The model under review builds one solid part; all positions refer to its coordinate system, in mm. Face numbers are marked on the shaded views. Round coordinates to 2 decimals unless told otherwise and drop trailing zeros. Write each loop counter-clockwise with the first axis right and the second up, starting at its lowest first coordinate (ties: lowest second). Pieces come first, ordered by that corner, then holes. Notation, with made-up numbers: (-22.5, 28) - (32.5, 28) arc R30 ccw to (32.5, 61) - close; hole circle Ø7 at (30, 40). An arc over 180 degrees is marked (long way). Use one line per item in the form item = value.
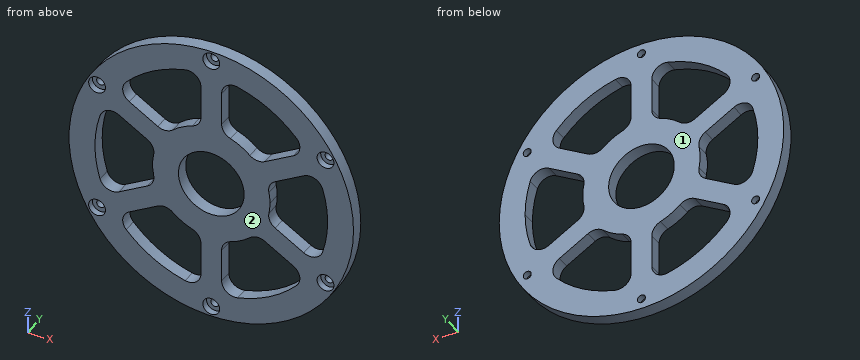
from build123d import *

# Parameters (mm, degrees)
SKETCH1_R           = 55
BOSS_EXTRUDE1_DEPTH = 5
SKETCH2_R           = 1.55
CUT_EXTRUDE1_DEPTH  = 6
SKETCH5_R           = 12.7
CUT_EXTRUDE4_DEPTH  = 6
CUT_EXTRUDE5_DEPTH  = 6
FILLET1_R           = 5
FILLET2_R           = 5
SKETCH8_R           = 3.25
CUT_EXTRUDE6_DEPTH  = 2.5
CIRPATTERN3_COUNT   = 6


with BuildPart() as part:
    # Sketch1 → Boss-Extrude1 (new body)
    with BuildSketch(Plane(origin=(0, 0, 0), x_dir=(1, 0, 0), z_dir=(0, 1, 0))):
        Circle(SKETCH1_R)
    extrude(amount=BOSS_EXTRUDE1_DEPTH)

    # Sketch2 → Cut-Extrude1 (cut, through all)
    with BuildSketch(Plane(origin=(0, 5, 0), x_dir=(1, 0, 0), z_dir=(0, 1, 0))):
        with Locations((0, 51)):
            Circle(SKETCH2_R)
        with Locations((44.167295593, 25.5)):
            Circle(SKETCH2_R)
        with Locations((44.167295593, -25.5)):
            Circle(SKETCH2_R)
        with Locations((0, -51)):
            Circle(SKETCH2_R)
        with Locations((-44.167295593, -25.5)):
            Circle(SKETCH2_R)
        with Locations((-44.167295593, 25.5)):
            Circle(SKETCH2_R)
    extrude(amount=-CUT_EXTRUDE1_DEPTH, mode=Mode.SUBTRACT)

    # Sketch5 → Cut-Extrude4 (cut, through all)
    with BuildSketch(Plane(origin=(0, 5, 0), x_dir=(1, 0, 0), z_dir=(0, 1, 0))):
        Circle(SKETCH5_R)
    extrude(amount=-CUT_EXTRUDE4_DEPTH, mode=Mode.SUBTRACT)

    # Sketch7 → Cut-Extrude5 (cut, through all)
    with BuildSketch(Plane(origin=(0, 5, 0), x_dir=(1, 0, 0), z_dir=(0, 1, 0))):
        with BuildLine():
            Line((-21.351162756, 7.708297411), (-40.816877772, 18.946833216))
            ThreePointArc((-40.816877772, 18.946833216), (-45, 0), (-40.816877772, -18.946833216))
            Line((-40.816877772, -18.946833216), (-21.351162756, -7.708297411))
            ThreePointArc((-21.351162756, -7.708297411), (-22.7, 0), (-21.351162756, 7.708297411))
        make_face()
        with BuildLine():
            Line((-17.351162756, -14.636500641), (-36.816877772, -25.875036446))
            ThreePointArc((-36.816877772, -25.875036446), (-22.5, -38.97114317), (-4, -44.821869662))
            Line((-4, -44.821869662), (-4, -22.344798052))
            ThreePointArc((-4, -22.344798052), (-11.35, -19.658776666), (-17.351162756, -14.636500641))
        make_face()
        with BuildLine():
            ThreePointArc((4, -44.821869662), (22.5, -38.97114317), (36.816877772, -25.875036446))
            Line((36.816877772, -25.875036446), (17.351162756, -14.636500641))
            ThreePointArc((17.351162756, -14.636500641), (11.35, -19.658776666), (4, -22.344798052))
            Line((4, -22.344798052), (4, -44.821869662))
        make_face()
        with BuildLine():
            ThreePointArc((45, 0), (43.941776818, 9.701559159), (40.816877772, 18.946833216))
            Line((40.816877772, 18.946833216), (21.351162756, 7.708297411))
            ThreePointArc((21.351162756, 7.708297411), (22.360248149, 3.912710406), (22.7, 0))
            ThreePointArc((22.7, 0), (22.360248149, -3.912710406), (21.351162756, -7.708297411))
            Line((21.351162756, -7.708297411), (40.816877772, -18.946833216))
            ThreePointArc((40.816877772, -18.946833216), (43.941776818, -9.701559159), (45, 0))
        make_face()
        with BuildLine():
            ThreePointArc((36.816877772, 25.875036446), (22.5, 38.97114317), (4, 44.821869662))
            Line((4, 44.821869662), (4, 22.344798052))
            ThreePointArc((4, 22.344798052), (11.35, 19.658776666), (17.351162756, 14.636500641))
            Line((17.351162756, 14.636500641), (36.816877772, 25.875036446))
        make_face()
        with BuildLine():
            Line((-4, 22.344798052), (-4, 44.821869662))
            ThreePointArc((-4, 44.821869662), (-22.5, 38.97114317), (-36.816877772, 25.875036446))
            Line((-36.816877772, 25.875036446), (-17.351162756, 14.636500641))
            ThreePointArc((-17.351162756, 14.636500641), (-11.35, 19.658776666), (-4, 22.344798052))
        make_face()
    extrude(amount=-CUT_EXTRUDE5_DEPTH, mode=Mode.SUBTRACT)

    # Fillet1
    fillet1_edges = [part.edges().sort_by_distance(p)[0] for p in [
        (-40.816877772, 2.5, -18.946833216),
        (-21.351162756, 2.5, -7.708297411),
        (-21.351162756, 2.5, 7.708297411),
        (-40.816877772, 2.5, 18.946833216),
    ]]
    fillet(fillet1_edges, radius=FILLET1_R)

    # Fillet2
    fillet2_edges = [part.edges().sort_by_distance(p)[0] for p in [
        (40.816877772, 2.5, 18.946833216),
        (21.351162756, 2.5, 7.708297411),
        (21.351162756, 2.5, -7.708297411),
        (40.816877772, 2.5, -18.946833216),
        (36.816877772, 2.5, -25.875036446),
        (17.351162756, 2.5, -14.636500641),
        (4, 2.5, -22.344798052),
        (4, 2.5, -44.821869662),
        (4, 2.5, 44.821869662),
        (4, 2.5, 22.344798052),
        (17.351162756, 2.5, 14.636500641),
        (36.816877772, 2.5, 25.875036446),
        (-36.816877772, 2.5, 25.875036446),
        (-17.351162756, 2.5, 14.636500641),
        (-4, 2.5, 22.344798052),
        (-4, 2.5, 44.821869662),
        (-4, 2.5, -44.821869662),
        (-4, 2.5, -22.344798052),
        (-17.351162756, 2.5, -14.636500641),
        (-36.816877772, 2.5, -25.875036446),
    ]]
    fillet(fillet2_edges, radius=FILLET2_R)

    # Sketch8 → Cut-Extrude6 (cut)
    with BuildSketch(Plane(origin=(0, 0, 0), x_dir=(1, 0, 0), z_dir=(0, 1, 0))):
        with Locations((0, 51)):
            Circle(SKETCH8_R)
    cut_extrude6 = extrude(amount=CUT_EXTRUDE6_DEPTH, mode=Mode.SUBTRACT)

    # CirPattern3: Cut-Extrude6 ×6 about axis
    cirpattern3_axis = Axis((0, 0, 0), (0, 1, 0))
    for i in range(1, CIRPATTERN3_COUNT):
        add(cut_extrude6.rotate(cirpattern3_axis, i * 360 / CIRPATTERN3_COUNT), mode=Mode.SUBTRACT)


solid = part.part
(1) Add section B-B on z = -1.5. Write out the cut boundary in (x, y) (3 decimals).
Geometry results:
outline = (-54.98, 0) - (-44.975, 0) - (-44.975, 5) - (-54.98, 5) - close; (-22.65, 0) - (-12.611, 0) - (-12.611, 5) - (-22.65, 5) - close; (12.611, 0) - (22.65, 0) - (22.65, 5) - (12.611, 5) - close; (44.975, 0) - (54.98, 0) - (54.98, 5) - (44.975, 5) - close
(2) To check wall thickness, follow L1, parallel to Z at x = 0, y = 4.05; L2, parallel to Z at x = 0, y = 0.7; L3, parallel to X at y = 1.7, z = -25.5. State the ranges of each line that lie inside material, in increasing order.
Geometry results:
L1 = -55 to -52.55, -49.45 to -12.7, 12.7 to 49.45, 52.55 to 55
L2 = -55 to -54.25, -47.75 to -12.7, 12.7 to 47.75, 54.25 to 55
L3 = -48.73 to -47.42, -40.92 to -33.92, -4.05 to 4.05, 33.92 to 40.92, 47.42 to 48.73
(3) Add section C-C on z = 51. Write out the cut boundary in (x, y).
Geometry results:
outline = (-20.59, 0) - (-3.25, 0) - (-3.25, 2.5) - (-1.55, 2.5) - (-1.55, 5) - (-20.59, 5) - close; (1.55, 2.5) - (3.25, 2.5) - (3.25, 0) - (20.59, 0) - (20.59, 5) - (1.55, 5) - close
(4) Add section A-A on x = 0. Write out the cut boundary in (y, z).
Geometry results:
outline = (0, -55) - (5, -55) - (5, -52.55) - (2.5, -52.55) - (2.5, -54.25) - (0, -54.25) - close; (0, -47.75) - (2.5, -47.75) - (2.5, -49.45) - (5, -49.45) - (5, -12.7) - (0, -12.7) - close; (0, 12.7) - (5, 12.7) - (5, 49.45) - (2.5, 49.45) - (2.5, 47.75) - (0, 47.75) - close; (0, 54.25) - (2.5, 54.25) - (2.5, 52.55) - (5, 52.55) - (5, 55) - (0, 55) - close
(5) Add section D-D on y = 3.4. Count the separate pieces of the cut face and the enclosed holes in it, then the cut area to 3 significant figures.
Geometry results:
separate_pieces = 1
enclosed_holes = 13
area = 5,410 mm2
(6) Insertion check: P1, Ø3, axis at x = 45, z = -24.5, coming from the -Y side; P2, Ø2.5, axis at x = 0, z = 51, coming from the +Y side; P3, Ø1.5, axis at y = 2, z = 33.5, coming from the -X side. Each pin has a flat end and moves straight along its axis. Give the tip position at first contact, or say it passes through.
Geometry results:
P1 = 2.5
P2 = through
P3 = -44.19
(7) The part is to be moulded in two halves that separate along Y. For the marked faces 1 and 2, say which applies: +Y half, -Y half, draft (parallel to the pull), parting line (faces both ways), or undercut.
Geometry results:
face_1 = +Y half
face_2 = -Y half
